Geometry: final body of the model. Coordinates: model frame, mm. A direction names the side the tool comes from. Round coordinates to 2 decimals unless told otherwise and drop trailing zeros. Loops run counter-clockwise (first coordinate to the right, second up) from the corner with the lowest first, then second, coordinate; pieces in that order, holes last. Notation, with made-up numbers: M -22.75,75.25 L -5.75,75.25 A31 cw -5.75,100.25 Z; hole C 30.5,25 d4. An arc over 180 degrees is marked long. Return JSON: item names as keys, results as strings.
from build123d import *

# Parameters (mm, degrees)
BOSS_EXTRUDE1_DEPTH      = 5
BOSS_EXTRUDE1_DEPTH_BACK = 5
SKETCH1_R                = 3
BOSS_EXTRUDE3_DEPTH      = 10
BOSS_EXTRUDE3_DEPTH_BACK = 10
SKETCH2_R                = 3
SHELL2_START             = -5
SHELL2_OUTLINE_R         = 2
SHELL2_DEPTH             = 10
SHELL2_START_2           = -10
SHELL2_2_OUTLINE_R       = 2
SHELL2_2_DEPTH           = 20


with BuildPart() as part:
    # Sketch1 → Boss-Extrude1 (new, two sides: drawn at the far end of the back side and taken through both)
    with BuildSketch(Plane(origin=(0, 0, 0), x_dir=(1, 0, 0), z_dir=(0, 1, 0)).offset(-BOSS_EXTRUDE1_DEPTH_BACK)):
        with Locations(Location((0, 0, 0), (0, 0, 270))):
            Circle(SKETCH1_R)
    extrude(amount=BOSS_EXTRUDE1_DEPTH + BOSS_EXTRUDE1_DEPTH_BACK)

    # Sketch2 → Boss-Extrude3 (add, two sides: drawn at the far end of the back side and taken through both)
    with BuildSketch(Plane(origin=(0, 0, 0), x_dir=(0, 0, -1), z_dir=(1, 0, 0)).offset(-BOSS_EXTRUDE3_DEPTH_BACK)):
        Circle(SKETCH2_R)
    extrude(amount=BOSS_EXTRUDE3_DEPTH + BOSS_EXTRUDE3_DEPTH_BACK)

    # Shell2: read off the stored shape, not the designer's step
    # Shell2 outline → Shell2 (cut)
    with BuildSketch(Plane(origin=(0, 0, 0), x_dir=(1, 0, 0), z_dir=(0, 1, 0)).offset(SHELL2_START)):
        Circle(SHELL2_OUTLINE_R)
    extrude(amount=SHELL2_DEPTH, mode=Mode.SUBTRACT)

    # Shell2 2 outline → Shell2 2 (cut)
    with BuildSketch(Plane.YZ.offset(SHELL2_START_2)):
        Circle(SHELL2_2_OUTLINE_R)
    extrude(amount=SHELL2_2_DEPTH, mode=Mode.SUBTRACT)


solid = part.part
Q1. Section query B-B (x = -1.5). Output: boundary loops of the cut face in (y, z), plus the area to 3 significant figures.
Determined:
{"outline": "M -5,-2.6 L -1.5,-2.6 A3 ccw 1.5,-2.6 L 5,-2.6 L 5,-1.32 L 1.5,-1.32 A2 cw -1.5,-1.32 L -5,-1.32 Z; M -5,1.32 L -1.5,1.32 A2 cw 1.5,1.32 L 5,1.32 L 5,2.6 L 1.5,2.6 A3 ccw -1.5,2.6 L -5,2.6 Z", "area": "24.3 mm^2"}
Q2. Material intervals for L1, parallel to Z at x = -5, y = 0; L2, parallel to X at y = 3.75, z = 0.3, sorted ascending.
Determined:
{"L1": "z = -3 to -2, 2 to 3", "L2": "x = -2.98 to -1.98, 1.98 to 2.98"}
Q3. Reachability of faces 1 (the flat face through (-1, 5, 2)), 2 (the cylindrical face through (0, -3, -3)), 3 (the cylindrical face through (-6.18, -1.15, -2.77)), 4 (the cylindrical face through (-1.8, 3, -2.4)) from +Z, -Z, +X, -X, +Y, -Y: full face, straight path, thin tool, end or side. Return the list, or none.
Determined:
{"face 1": "+Z, -Z, +X, -X, +Y", "face 2": "-Y", "face 3": "-X", "face 4": "+Y"}
Q4. Section query A-A (z = 0). Output: boundary loops of the cut face in (x, y), plus the area to 3 significant figures.
Determined:
{"outline": "M -10,-3 L -3,-3 L -3,-5 L -2,-5 L -2,-2 L -10,-2 Z; M -10,2 L -2,2 L -2,5 L -3,5 L -3,3 L -10,3 Z; M 2,-5 L 3,-5 L 3,-3 L 10,-3 L 10,-2 L 2,-2 Z; M 2,2 L 10,2 L 10,3 L 3,3 L 3,5 L 2,5 Z", "area": "40.0 mm^2"}
Q5. Pull-direction query (Y, two-part tool) for faces 5 (the cylindrical face through (1.847, 3.021, 0.766)), 6 (the cylindrical face through (6.04, -1.15, -2.77)), 7 (the cylindrical face through (-6, -2, 0)); classes: pulls with the +Y half, pulls with the -Y half, needs draft (parallel to the pull), parting line crosses it, or undercut.
Determined:
{"face 5": "needs draft", "face 6": "parting line crosses it", "face 7": "undercut"}
Q6. Pin query (flat end, axial travel): pin 1 (1 mm diameter, centred on x = -3.5, z = 1, fed in from -Y); pin 2 (1.5 mm diameter, centred on x = -2, y = -1.5, fed in from -Z); pin 3 (1 mm diameter, centred on x = 1.5, y = 2, fed in from -Z). Return the tip coordinate at first contact, or that it passes through.
Determined:
{"pin 1": "stops at y = -2.96", "pin 2": "stops at z = -2.9", "pin 3": "stops at z = -2.83"}
Q7. Section query D-D (x = 3.5). Output: boundary loops of the cut face in (y, z), plus the area to 3 significant figures.
Determined:
{"outline": "C 0,0 d6; hole C 0,0 d4", "area": "15.7 mm^2"}
Q8. Section query C-C (y = -0.5). Output: boundary loops of the cut face in (x, z), plus the area to 3 significant figures.
Determined:
{"outline": "M -10,-2.96 L -0.5,-2.96 A3 ccw 0.5,-2.96 L 10,-2.96 L 10,-1.94 L 0.5,-1.94 A2 cw -0.5,-1.94 L -10,-1.94 Z; M -10,1.94 L -0.5,1.94 A2 cw 0.5,1.94 L 10,1.94 L 10,2.96 L 0.5,2.96 A3 ccw -0.5,2.96 L -10,2.96 Z", "area": "40.8 mm^2"}
